Model file for the job. Use its own axes, mm. A direction names the side the tool comes from. Coordinates: 2 decimals unless noted, no trailing zeros. Order: outer loops, then holes, each group sorted by start corner. A loop starts at its lowest first (then second) coordinate and runs counter-clockwise, first axis right, second up. Notation, with made-up numbers: (-24, -20.75) -> (0, -20.75) arc R10 cw to (0, -9.75) -> close; hole circle Ø5 at (-0.5, -29). An arc over 180 degrees is marked (long way). Write item = value, one per line. Start each with the question number.
Q1. Flat gauge pins, fed straight in: pin 1 (6 mm diameter, centred on y = 89, z = 12, fed in from -X); pin 2 (8 mm diameter, centred on x = 357.5, z = 232.5, fed in from +Y); pin 3 (2.5 mm diameter, centred on y = 90, z = 204, fed in from -X). Where does each tip first touch, or does it go through?
Q2. Cut at A-A, the plane z = -187.5. List the corners of the cut face in (x, y), plus the area to 3 significant figures.
Q3. Mould opens along Z. For faces 4 (the face through (-6, 49, -340)), 5 (the face through (-450, 39, 5)), 6 (the face through (-42, 98, 82)), 7 (the face through (-402.788, 79.507, -238.453)) say: +Z half, -Z half, draft (parallel to the pull), parting line (faces both ways), or undercut.
Q4. Wall check: line 1 (Z direction, x = -290.5, y = 40); line 2 (Z direction, x = 332, y = 90); line 3 (Y direction, x = -131, z = 0). Give the ranges that are in metal, low to high. Write a range as from..to.
Q5. 3-axis set-ups, long thin cutter, end or side, ignore diameter. For faces 1 (the face through (335.5, 90, 5)), 2 (the face through (-398, 79, -250)), 3 (the face through (-394, 80, -5)): which of +Z, -Z, +X, -X, +Y, -Y reach the whole face in a straight line?
from build123d import *

# Parameters (mm, degrees)
SKETCH_1_W                    = 900
SKETCH_1_H                    = 680
EXTRUDE_1_DEPTH               = 80
SKETCH_2_W                    = 671
SKETCH_2_H                    = 680
EXTRUDE_2_DEPTH               = 20
SKETCH_4_W                    = 312
SKETCH_4_H                    = 112
CUT_EXTRUDE_1_DEPTH           = 2
HOLE_WIZARD_M5_1_D            = 4.2
HOLE_WIZARD_M5_1_DEPTH        = 9
HOLE_WIZARD_M5_1_TIP          = 1.2618073
HOLE_WIZARD_M5_2_D            = 4.2
HOLE_WIZARD_M5_3_D            = 4.2
SKETCH_15_R                   = 12.5
CUT_EXTRUDE_2_DEPTH           = 1
HOLE_WIZARD_M3_5_1_AT_2_COUNT = 2
HOLE_WIZARD_M3_5_1_AT_2_PITCH = 136
HOLE_WIZARD_M3_5_1_AT_3_COUNT = 2
HOLE_WIZARD_M3_5_1_AT_3_PITCH = 272
HOLE_WIZARD_M3_5_1_AT_4_COUNT = 2
HOLE_WIZARD_M3_5_1_AT_4_PITCH = 408


with BuildPart() as part:
    # 草图1 → 凸台-拉伸1 (new body)
    with BuildSketch(Plane(origin=(0, 0, 0), x_dir=(1, 0, 0), z_dir=(0, 1, 0))):
        Rectangle(SKETCH_1_W, SKETCH_1_H)
    extrude(amount=EXTRUDE_1_DEPTH)

    # 草图2 → 凸台-拉伸2 (add)
    with BuildSketch(Plane(origin=(0, 80, 0), x_dir=(1, 0, 0), z_dir=(0, 1, 0))):
        Rectangle(SKETCH_2_W, SKETCH_2_H)
    extrude(amount=EXTRUDE_2_DEPTH)

    # 草图4 → 切除-拉伸1 (cut)
    with BuildSketch(Plane(origin=(0, 100, 0), x_dir=(1, 0, 0), z_dir=(0, 1, 0))):
        with Locations((-40, -83)):
            Rectangle(SKETCH_4_W, SKETCH_4_H)
    extrude(amount=-CUT_EXTRUDE_1_DEPTH, mode=Mode.SUBTRACT)

    # M5 螺纹孔1
    with Locations(Plane(origin=(0, 100, 0), x_dir=(1, 0, 0), z_dir=(0, 1, 0))):
        with Locations((-180, -83), (-40, -43), (-40, -123), (100, -83)):
            Hole(HOLE_WIZARD_M5_1_D / 2, depth=HOLE_WIZARD_M5_1_DEPTH)
            with Locations((0, 0, -(HOLE_WIZARD_M5_1_DEPTH + HOLE_WIZARD_M5_1_TIP / 2))):  # 118° drill point
                Cone(0, HOLE_WIZARD_M5_1_D / 2, HOLE_WIZARD_M5_1_TIP, mode=Mode.SUBTRACT)

    # M5 螺纹孔2 (through all)
    with Locations(Plane.XY.offset(340)):
        with Locations((0, 40)):
            Hole(HOLE_WIZARD_M5_2_D / 2)

    # M5 螺纹孔3 (through all)
    with Locations(Plane.ZY.offset(450)):
        with Locations((0, 40)):
            Hole(HOLE_WIZARD_M5_3_D / 2)

    # 草图15 → 切除-拉伸2 (cut)
    with BuildSketch(Plane(origin=(0, 80, 0), x_dir=(1, 0, 0), z_dir=(0, 1, 0))):
        with Locations(Location((-398, 250, 0), (0, 0, 270))):
            Circle(SKETCH_15_R)
    extrude(amount=-CUT_EXTRUDE_2_DEPTH, mode=Mode.SUBTRACT)

    # 草图19 → M3.5 螺纹孔1 (revolve, cut)
    with BuildSketch(Plane(origin=(-335.5, 90, -204), x_dir=(0, 0, 1), z_dir=(0, 1, 0))):
        Polygon((0, 0), (0, 8.271247898), (1.45, 7.4), (1.45, 0), align=None)
    hole_wizard_m3_5_1 = revolve(axis=Axis((-341.85, 90, -204), (1, 0, 0)), mode=Mode.SUBTRACT)

    # M3.5 螺纹孔1 at 2: M3.5 螺纹孔1 ×2
    with Locations(*[(0, 0, i * HOLE_WIZARD_M3_5_1_AT_2_PITCH) for i in range(1, HOLE_WIZARD_M3_5_1_AT_2_COUNT)]):
        add(hole_wizard_m3_5_1, mode=Mode.SUBTRACT)

    # M3.5 螺纹孔1 at 3: M3.5 螺纹孔1 ×2
    with Locations(*[(0, 0, i * HOLE_WIZARD_M3_5_1_AT_3_PITCH) for i in range(1, HOLE_WIZARD_M3_5_1_AT_3_COUNT)]):
        add(hole_wizard_m3_5_1, mode=Mode.SUBTRACT)

    # M3.5 螺纹孔1 at 4: M3.5 螺纹孔1 ×2
    with Locations(*[(0, 0, i * HOLE_WIZARD_M3_5_1_AT_4_PITCH) for i in range(1, HOLE_WIZARD_M3_5_1_AT_4_COUNT)]):
        add(hole_wizard_m3_5_1, mode=Mode.SUBTRACT)

    # 镜向1: M3.5 螺纹孔1 across plane
    add(hole_wizard_m3_5_1.mirror(Plane(origin=(0, 0, 0), x_dir=(0, 0, 1), z_dir=(1, 0, 0))), mode=Mode.SUBTRACT)

    # 镜向1 copy 1 sketch → 镜向1 copy 1 (revolve, cut)
    with BuildSketch(Plane(origin=(335.5, 90, -68), x_dir=(0, 0, 1), z_dir=(0, 1, 0))):
        Polygon((0, 0), (0, -8.271247898), (1.45, -7.4), (1.45, 0), align=None)
    revolve(axis=Axis((341.85, 90, -68), (1, 0, 0)), mode=Mode.SUBTRACT)

    # 镜向1 copy 2 sketch → 镜向1 copy 2 (revolve, cut)
    with BuildSketch(Plane(origin=(335.5, 90, 68), x_dir=(0, 0, 1), z_dir=(0, 1, 0))):
        Polygon((0, 0), (0, -8.271247898), (1.45, -7.4), (1.45, 0), align=None)
    revolve(axis=Axis((341.85, 90, 68), (1, 0, 0)), mode=Mode.SUBTRACT)

    # 镜向1 copy 3 sketch → 镜向1 copy 3 (revolve, cut)
    with BuildSketch(Plane(origin=(335.5, 90, 204), x_dir=(0, 0, 1), z_dir=(0, 1, 0))):
        Polygon((0, 0), (0, -8.271247898), (1.45, -7.4), (1.45, 0), align=None)
    revolve(axis=Axis((341.85, 90, 204), (1, 0, 0)), mode=Mode.SUBTRACT)


solid = part.part
Here are the results:
q1.pin_1 = -335.5
q1.pin_2 = 80
q1.pin_3 = -327.98
q2.outline = (-450, 0) -> (450, 0) -> (450, 80) -> (335.5, 80) -> (335.5, 100) -> (-335.5, 100) -> (-335.5, 80) -> (-450, 80) -> close; hole circle Ø4.2 at (0, 40)
q2.area = 85,400 mm²
q3.face_4 = -Z half
q3.face_5 = draft
q3.face_6 = undercut
q3.face_7 = undercut
q4.line_1 = -340..-2.1, 2.1..340
q4.line_2 = -340..-205.45, -202.55..-69.45, -66.55..66.55, 69.45..202.55, 205.45..340
q4.line_3 = 0..37.9, 42.1..100
q5.face_1 = +Z, -Z, +X, +Y
q5.face_2 = +Y
q5.face_3 = +Z, -Z, -X, +Y
